from build123d import *

# Parameters (mm, degrees)
F0_W     = 44
F0_H     = 47
F0_R     = 1.5
F0_W_2   = 14.9
F0_H_2   = 8
F0_W_3   = 8
F0_H_3   = 10.5
F0_W_4   = 23.4
F0_H_4   = 16
F0_R_2   = 1.6
F0_W_5   = 2.5
F0_H_5   = 2.5
F0_W_6   = 1
F0_H_6   = 1
F1_DEPTH = 1.6
F2_DEPTH = 24.8
F3_DEPTH = 10.2
F4_DEPTH = 6
F5_DEPTH = 2
F6_DEPTH = 6


with BuildPart() as f1:
    # F0 (on Top) → F1 (new body)
    with BuildSketch(Plane.XY):
        Rectangle(F0_W, F0_H)
        with Locations((-19.05, -17.45)):
            Circle(F0_R, mode=Mode.SUBTRACT)
        with Locations((-9.0953609079, -14.8641939312)):
            Rectangle(F0_W_2, F0_H_2, mode=Mode.SUBTRACT)
        with Locations((-16.8999998868, -4.2141940668)):
            Rectangle(F0_W_3, F0_H_3, mode=Mode.SUBTRACT)
        Polygon((4.6191942506, -18.8641939312), (2.1191942506, -18.8641939312), (2.1191942506, -16.3641939312), (4.6191942506, -16.3641939312), (7.1191942506, -16.3641939312), (9.6191942506, -16.3641939312), (12.1191942506, -16.3641939312), (12.1191942506, -18.8641939312), (9.6191942506, -18.8641939312), (7.1191942506, -18.8641939312), align=None, mode=Mode.SUBTRACT)
        with Locations((18.9, -17.5)):
            Circle(F0_R, mode=Mode.SUBTRACT)
        with Locations((17.1648499519, -4.2141940668)):
            Rectangle(F0_W_3, F0_H_3, mode=Mode.SUBTRACT)
        with Locations((-18.8, 20.55)):
            Circle(F0_R, mode=Mode.SUBTRACT)
        with Locations((0, 15)):
            Rectangle(F0_W_4, F0_H_4, mode=Mode.SUBTRACT)
        with Locations((18.8, 20.55)):
            Circle(F0_R, mode=Mode.SUBTRACT)
        with Locations((0, 15)):
            Rectangle(F0_W_4, F0_H_4)
        with Locations((-9.0953609079, -14.8641939312)):
            Rectangle(F0_W_2, F0_H_2)
        with Locations((-12.8203609079, -14.8641939312)):
            Circle(F0_R_2, mode=Mode.SUBTRACT)
        with Locations((-9.0953609079, -14.8641939312)):
            Circle(F0_R_2, mode=Mode.SUBTRACT)
        with Locations((-5.3703609079, -14.8641939312)):
            Circle(F0_R_2, mode=Mode.SUBTRACT)
        with Locations((17.1648499519, -4.2141940668)):
            Rectangle(F0_W_3, F0_H_3)
        with Locations((17.1648499519, -6.8391940668)):
            Circle(F0_R_2, mode=Mode.SUBTRACT)
        with Locations((17.1648499519, -1.5891940668)):
            Circle(F0_R_2, mode=Mode.SUBTRACT)
        with Locations((-16.8999998868, -4.2141940668)):
            Rectangle(F0_W_3, F0_H_3)
        with Locations((-16.8999998868, -6.8391940668)):
            Circle(F0_R_2, mode=Mode.SUBTRACT)
        with Locations((-16.8999998868, -1.5891940668)):
            Circle(F0_R_2, mode=Mode.SUBTRACT)
        with Locations((-16.8999998868, -1.5891940668)):
            Circle(F0_R_2)
        with Locations((-16.8999998868, -6.8391940668)):
            Circle(F0_R_2)
        with Locations((-12.8203609079, -14.8641939312)):
            Circle(F0_R_2)
        with Locations((-9.0953609079, -14.8641939312)):
            Circle(F0_R_2)
        with Locations((-5.3703609079, -14.8641939312)):
            Circle(F0_R_2)
        with Locations((17.1648499519, -6.8391940668)):
            Circle(F0_R_2)
        with Locations((17.1648499519, -1.5891940668)):
            Circle(F0_R_2)
        with Locations((3.3691942506, -17.6141939312)):
            Rectangle(F0_W_5, F0_H_5)
        with Locations((3.3691942506, -17.6141939312)):
            Rectangle(F0_W_6, F0_H_6, mode=Mode.SUBTRACT)
        with Locations((5.8691942506, -17.6141939312)):
            Rectangle(F0_W_5, F0_H_5)
        with Locations((5.8691942506, -17.6141939312)):
            Rectangle(F0_W_6, F0_H_6, mode=Mode.SUBTRACT)
        with Locations((8.3691942506, -17.6141939312)):
            Rectangle(F0_W_5, F0_H_5)
        with Locations((8.3691942506, -17.6141939312)):
            Rectangle(F0_W_6, F0_H_6, mode=Mode.SUBTRACT)
        with Locations((10.8691942506, -17.6141939312)):
            Rectangle(F0_W_5, F0_H_5)
        with Locations((10.8691942506, -17.6141939312)):
            Rectangle(F0_W_6, F0_H_6, mode=Mode.SUBTRACT)
        with Locations((3.3691942506, -17.6141939312)):
            Rectangle(F0_W_6, F0_H_6)
        with Locations((5.8691942506, -17.6141939312)):
            Rectangle(F0_W_6, F0_H_6)
        with Locations((10.8691942506, -17.6141939312)):
            Rectangle(F0_W_6, F0_H_6)
        with Locations((8.3691942506, -17.6141939312)):
            Rectangle(F0_W_6, F0_H_6)
    extrude(amount=-F1_DEPTH)

    # F0 (on Top) → F2 (join)
    with BuildSketch(Plane.XY):
        with Locations((0, 15)):
            Rectangle(F0_W_4, F0_H_4)
    extrude(amount=F2_DEPTH)

    # F0 (on Top) → F3 (join)
    with BuildSketch(Plane.XY):
        with Locations((-16.8999998868, -4.2141940668)):
            Rectangle(F0_W_3, F0_H_3)
        with Locations((-16.8999998868, -6.8391940668)):
            Circle(F0_R_2, mode=Mode.SUBTRACT)
        with Locations((-16.8999998868, -1.5891940668)):
            Circle(F0_R_2, mode=Mode.SUBTRACT)
        with Locations((-9.0953609079, -14.8641939312)):
            Rectangle(F0_W_2, F0_H_2)
        with Locations((-12.8203609079, -14.8641939312)):
            Circle(F0_R_2, mode=Mode.SUBTRACT)
        with Locations((-9.0953609079, -14.8641939312)):
            Circle(F0_R_2, mode=Mode.SUBTRACT)
        with Locations((-5.3703609079, -14.8641939312)):
            Circle(F0_R_2, mode=Mode.SUBTRACT)
        with Locations((17.1648499519, -4.2141940668)):
            Rectangle(F0_W_3, F0_H_3)
        with Locations((17.1648499519, -6.8391940668)):
            Circle(F0_R_2, mode=Mode.SUBTRACT)
        with Locations((17.1648499519, -1.5891940668)):
            Circle(F0_R_2, mode=Mode.SUBTRACT)
    extrude(amount=F3_DEPTH)

    # F0 (on Top) → F4 (join)
    with BuildSketch(Plane.XY):
        with Locations((-16.8999998868, -1.5891940668)):
            Circle(F0_R_2)
        with Locations((-16.8999998868, -6.8391940668)):
            Circle(F0_R_2)
        with Locations((-12.8203609079, -14.8641939312)):
            Circle(F0_R_2)
        with Locations((-9.0953609079, -14.8641939312)):
            Circle(F0_R_2)
        with Locations((-5.3703609079, -14.8641939312)):
            Circle(F0_R_2)
        with Locations((17.1648499519, -6.8391940668)):
            Circle(F0_R_2)
        with Locations((17.1648499519, -1.5891940668)):
            Circle(F0_R_2)
    extrude(amount=F4_DEPTH)

    # F0 (on Top) → F5 (join)
    with BuildSketch(Plane.XY):
        with Locations((3.3691942506, -17.6141939312)):
            Rectangle(F0_W_5, F0_H_5)
        with Locations((3.3691942506, -17.6141939312)):
            Rectangle(F0_W_6, F0_H_6, mode=Mode.SUBTRACT)
        with Locations((5.8691942506, -17.6141939312)):
            Rectangle(F0_W_5, F0_H_5)
        with Locations((5.8691942506, -17.6141939312)):
            Rectangle(F0_W_6, F0_H_6, mode=Mode.SUBTRACT)
        with Locations((8.3691942506, -17.6141939312)):
            Rectangle(F0_W_5, F0_H_5)
        with Locations((8.3691942506, -17.6141939312)):
            Rectangle(F0_W_6, F0_H_6, mode=Mode.SUBTRACT)
        with Locations((10.8691942506, -17.6141939312)):
            Rectangle(F0_W_5, F0_H_5)
        with Locations((10.8691942506, -17.6141939312)):
            Rectangle(F0_W_6, F0_H_6, mode=Mode.SUBTRACT)
    extrude(amount=F5_DEPTH)

    # F0 (on Top) → F6 (join)
    with BuildSketch(Plane.XY):
        with Locations((3.3691942506, -17.6141939312)):
            Rectangle(F0_W_6, F0_H_6)
        with Locations((5.8691942506, -17.6141939312)):
            Rectangle(F0_W_6, F0_H_6)
        with Locations((8.3691942506, -17.6141939312)):
            Rectangle(F0_W_6, F0_H_6)
        with Locations((10.8691942506, -17.6141939312)):
            Rectangle(F0_W_6, F0_H_6)
    extrude(amount=F6_DEPTH)


solid = f1.part
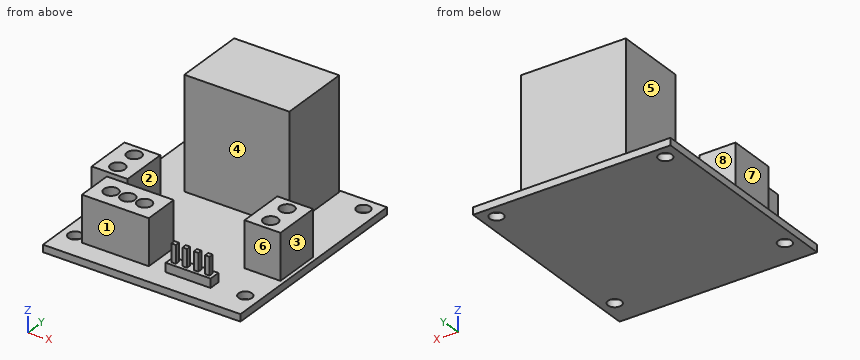
Geometry check sheet. Reference: the model listing, model coordinates, mm. Face numbers are marked on the shaded views. A direction names the side the tool comes from. Coordinates: 2 decimals unless noted, no trailing zeros. Order: outer loops, then holes, each group sorted by start corner. A loop starts at its lowest first (then second) coordinate and runs counter-clockwise, first axis right, second up. Notation, with made-up numbers: (57, -40) - (63, -40) arc R11 ccw to (63, -23) - close; hole circle Ø10 at (-11.5, 25). An arc over 180 degrees is marked (long way). One line per item, written item: value.
(1) Sectioned sample at C-C (y = 11). Enter the section's corners in (x, z), and give its area (3 significant figures).
Data:
outline: (-22, -1.6) - (22, -1.6) - (22, 0) - (11.7, 0) - (11.7, 24.8) - (-11.7, 24.8) - (-11.7, 0) - (-22, 0) - close
area: 651 mm^2
(2) Sectioned sample at D-D (z = 11.25). Enter the section's corners in (x, y), and give its area (3 significant figures).
Data:
outline: (-11.7, 7) - (11.7, 7) - (11.7, 23) - (-11.7, 23) - close
area: 374 mm^2
(3) Sectioned sample at B-B (x = 18). Enter the section's corners in (y, z), and give its area (3 significant figures).
Data:
outline: (-23.5, -1.6) - (-18.7, -1.6) - (-18.7, 0) - (-23.5, 0) - close; (-16.3, -1.6) - (19.28, -1.6) - (19.28, 0) - (1.04, 0) - (1.04, 10.2) - (-0.22, 10.2) - (-0.22, 6) - (-2.95, 6) - (-2.95, 10.2) - (-5.47, 10.2) - (-5.47, 6) - (-8.2, 6) - (-8.2, 10.2) - (-9.46, 10.2) - (-9.46, 0) - (-16.3, 0) - close; (21.82, -1.6) - (23.5, -1.6) - (23.5, 0) - (21.82, 0) - close
area: 151 mm^2
(4) Depth check by flat-ended pin: pin 1 Ø2.5 at (y, z) = (-13.5, 3.5) entering from -X; pin 2 Ø1 at (x, z) = (13.5, 10.5) entering from -Y; pin 3 Ø9 at (x, z) = (-15.5, 6) entering from -Y. Enter the tip coordinate at first touch or a pass-through.
Data:
pin 1: stops at x = -16.55
pin 2: stops at y = -9.46
pin 3: stops at y = -18.86
(5) Thickness scan on probe 1 along Y at (x, z) = (-16.9, 8.4); probe 2 along Y at (x, z) = (-8, 7.5); probe 3 along Z at (x, y) = (0, -2). Record the ranges inside material, lowest first. Write a range as from..to.
Data:
probe 1: y = -9.46..-8.44, -5.24..-3.19, 0.01..1.04
probe 2: y = -18.86..-16.03, -13.7..-10.86, 7..23
probe 3: z = -1.6..0
(6) Release check for a two-part mould opening along X. For the marked faces 1, 2 and 3 record: +X half, -X half, draft (parallel to the pull), parting line (faces both ways), or undercut.
Data:
face 1: draft
face 2: undercut
face 3: +X half
(7) Access from +Z, -Z, +X, -X, +Y, -Y to the whole of each face (thin tool, end or side, straight path). Record for the marked faces 4, 5, 6, 7 and 8.
Data:
face 4: +Z, +X, -X
face 5: +Z, -X, +Y
face 6: +Z, +X, -X, -Y
face 7: +Z, -X, +Y, -Y
face 8: +Z, +X, -X, +Y
(8) Sectioned sample at A-A (y = 20.55). Enter the section's corners in (x, z), and give its area (3 significant figures).
Data:
outline: (-22, -1.6) - (-20.3, -1.6) - (-20.3, 0) - (-22, 0) - close; (-17.3, -1.6) - (17.3, -1.6) - (17.3, 0) - (11.7, 0) - (11.7, 24.8) - (-11.7, 24.8) - (-11.7, 0) - (-17.3, 0) - close; (20.3, -1.6) - (22, -1.6) - (22, 0) - (20.3, 0) - close
area: 641 mm^2
